Here's how the part is built. I have some questions about the finished solid (model axes, mm). A direction names the side the tool comes from. Coordinates: 2 decimals unless noted, no trailing zeros. Write each loop counter-clockwise with the first axis right and the second up, starting at its lowest first coordinate (ties: lowest second). Pieces come first, ordered by that corner, then holes. Notation, with made-up numbers: (-32.5, 86) - (9.5, 86) arc R21 cw to (9.5, 95) - close; hole circle Ø5 at (-5.5, 7). An arc over 180 degrees is marked (long way). Answer in a Markdown table with one row per item. Add a question column.
Item 1: Imagine slicing it at D-D (y = -52.5). Please give me the cut outline in (x, z).
Item 2: Imagine slicing it at A-A (z = 17.5). Please give me the cut outline in (x, y).
Item 3: We'd pull the mould along X, two halves only. Please class faces 6 (the face through (-35, -45, 5)), 7 (the face through (40, -64, 10)), 8 (the face through (-16, 40, 10)): +X half, -X half, draft (parallel to the pull), parting line (faces both ways), or undercut.
Item 4: Imagine slicing it at C-C (y = -31.5). Please give me the cut outline in (x, z), plus the area to 3 significant figures.
Item 5: Imagine slicing it at B-B (x = -4). Please give me the cut outline in (y, z), plus the area to 3 significant figures.
Item 6: If I drill on probe 1 along X at (y, z) = (-29.5, 27); probe 2 along X at (y, z) = (-39.5, 10.75); probe 3 along Y at (x, z) = (15, 26.5), over which ranges is the centre line in solid material (lowest first)? Write a range as from..to.
Item 7: Which directions (+Z, -Z, +X, -X, +Y, -Y) give clear straight access to the entire face, cutting with the end or side of a thin tool? Please do faces 1 (the face through (-28.1, -35, 9)), 2 (the face through (-1, -68, 5)), 3 (the face through (27, -54.5, 15)), 4 (the face through (-11.1, 40, 15)), 5 (the face through (16, -20, 15)).
Item 8: I'm going to push flat-ended pins straight in: pin 1 (4 mm diameter, centred on x = 37, z = 17, fed in from -Y); pin 2 (3 mm diameter, centred on y = -23, z = 2.5, fed in from -X); pin 3 (4.5 mm diameter, centred on y = -39, z = 3, fed in from +X). Where does each tip first touch, or does it pass through?
from build123d import *

# Parameters (mm, degrees)
PAD_DEPTH       = 30
POCKET_DEPTH    = 22
POCKET001_DEPTH = 6.9
SKETCH003_W     = 25.3
SKETCH003_H     = 23
SKETCH003_W_2   = 14.2
SKETCH003_H_2   = 27
POCKET002_DEPTH = 30
SKETCH004_W     = 10
SKETCH004_H     = 10
POCKET003_DEPTH = 50
POCKET004_DEPTH = 20


with BuildPart() as part:
    # Sketch → Pad (new body)
    with BuildSketch(Plane.XY):
        with BuildLine():
            Line((-35, 44.027333), (-35, 37.027333))
            Line((-35, 37.027333), (24.9, 37.027333))
            ThreePointArc((34.9, 26.230332), (32.268481, 33.822479), (24.9, 37.027333))
            Line((34.9, -9.769668), (34.9, 26.230332))
            ThreePointArc((24.9, -20), (32.053765, -16.990108), (34.9, -9.769668))
            Line((24.9, -20), (-28.1, -20))
            Line((-28.1, -27), (-28.1, -20))
            Line((-35, -27), (-28.1, -27))
            Line((-35, -27), (-35, -62))
            Line((-35, -62), (-35, -74.5))
            Line((-35, -74.5), (-1, -74.5))
            Line((-1, -74.5), (-1, -62))
            Line((-1, -62), (16.9, -62))
            Line((16.9, -62), (29.4, -74.5))
            Line((29.4, -74.5), (54.4, -74.5))
            Line((54.4, -74.5), (54.4, -49.5))
            Line((54.4, -49.5), (41.9, -37))
            Line((41.9, 10.027333), (41.9, -37))
            Line((54.4, 10.027333), (41.9, 10.027333))
            Line((54.4, 44.027333), (54.4, 10.027333))
            Line((41.9, 44.027333), (54.4, 44.027333))
            Line((41.9, 44.027333), (-35, 44.027333))
        make_face()
    extrude(amount=PAD_DEPTH)

    # Sketch001 → Pocket (cut)
    with BuildSketch(Plane.XY.offset(4)):
        Polygon((-28.1, -20), (-28.1, -58.5), (12.2, -58.5), (12.2, -20), (-18.1, -20), (-18.1, -13.5), (-24.1, -13.5), (-24.1, -20), align=None)
    extrude(amount=POCKET_DEPTH, mode=Mode.SUBTRACT)

    # Sketch002 → Pocket001 (cut)
    with BuildSketch(Plane.YZ.offset(-35)):
        Polygon((-27, 26.185834), (-27, 14.185834), (-37, 14.185834), (-47, 4), (-57, 4), (-57, 26.185834), align=None)
    extrude(amount=POCKET001_DEPTH, mode=Mode.SUBTRACT)

    # Sketch003 → Pocket002 (cut)
    with BuildSketch(Plane.XY):
        with Locations((-7.95, -39)):
            Rectangle(SKETCH003_W, SKETCH003_H)
        with Locations((26.8, -41)):
            Rectangle(SKETCH003_W_2, SKETCH003_H_2)
    extrude(amount=POCKET002_DEPTH, mode=Mode.SUBTRACT)

    # Sketch004 → Pocket003 (cut)
    with BuildSketch(Plane.XZ):
        with Locations((-16.1, 15)):
            Rectangle(SKETCH004_W, SKETCH004_H)
    extrude(amount=-POCKET003_DEPTH, mode=Mode.SUBTRACT)

    # Sketch005 → Pocket004 (cut)
    with BuildSketch(Plane.XY.offset(10)):
        Polygon((54.4, -61.416298), (54.4, -74.5), (-35, -74.5), (-35, -62), (41.9, -62), (41.9, 44.9), (54.4, 44.9), align=None)
    extrude(amount=POCKET004_DEPTH, mode=Mode.SUBTRACT)


solid = part.part
Here are the results:
| question | item | result |
|---|---|---|
| 1 | outline | (-35, 0) - (19.7, 0) - (19.7, 30) - (-35, 30) - (-35, 26.19) - (-28.1, 26.19) - (-28.1, 26) - (12.2, 26) - (12.2, 4) - (-35, 4) - close; (33.9, 0) - (54.4, 0) - (54.4, 10) - (41.9, 10) - (41.9, 30) - (33.9, 30) - close |
| 2 | outline | (-35, -62) - (41.9, -62) - (41.9, 44.03) - (-11.1, 44.03) - (-11.1, 37.03) - (24.9, 37.03) arc R10 cw to (34.9, 26.23) - (34.9, -9.77) arc R10 cw to (24.9, -20) - (12.2, -20) - (12.2, -58.5) - (-28.1, -58.5) - (-28.1, -57) - (-35, -57) - close; (-35, 37.03) - (-21.1, 37.03) - (-21.1, 44.03) - (-35, 44.03) - close; hole (19.7, -54.5) - (33.9, -54.5) - (33.9, -27.5) - (19.7, -27.5) - close |
| 3 | face 6 | -X half |
| 3 | face 7 | draft |
| 3 | face 8 | undercut |
| 4 | outline | (-35, 0) - (-20.6, 0) - (-20.6, 4) - (-28.1, 4) - (-28.1, 14.19) - (-35, 14.19) - close; (-35, 26.19) - (-28.1, 26.19) - (-28.1, 26) - (-20.6, 26) - (-20.6, 30) - (-35, 30) - close; (4.7, 0) - (19.7, 0) - (19.7, 30) - (4.7, 30) - (4.7, 26) - (12.2, 26) - (12.2, 4) - (4.7, 4) - close; (33.9, 0) - (41.9, 0) - (41.9, 30) - (33.9, 30) - close |
| 4 | area | 709 mm2 |
| 5 | outline | (-74.5, 0) - (-50.5, 0) - (-50.5, 4) - (-58.5, 4) - (-58.5, 26) - (-50.5, 26) - (-50.5, 30) - (-62, 30) - (-62, 10) - (-74.5, 10) - close; (-27.5, 0) - (-20, 0) - (-20, 4) - (-27.5, 4) - close; (-27.5, 26) - (-20, 26) - (-20, 30) - (-27.5, 30) - close; (37.03, 0) - (44.03, 0) - (44.03, 30) - (37.03, 30) - close |
| 5 | area | 564 mm2 |
| 6 | probe 1 | x = -35..-20.6, 4.7..19.7, 33.9..41.9 |
| 6 | probe 2 | x = -35..-28.1, 12.2..19.7, 33.9..41.9 |
| 6 | probe 3 | y = -62..-20, 37.03..44.03 |
| 7 | face 1 | none |
| 7 | face 2 | +Z, -Z, -Y |
| 7 | face 3 | +Z, -Z |
| 7 | face 4 | +Y |
| 7 | face 5 | +Z, -Z, -X |
| 8 | pin 1 | stops at y = -62 |
| 8 | pin 2 | stops at x = -28.1 |
| 8 | pin 3 | stops at x = 46.15 |
